Work out the finished part from the listing and answer in its coordinate system (mm). A direction names the side the tool comes from. Round coordinates to 2 decimals unless told otherwise and drop trailing zeros. Write each loop counter-clockwise with the first axis right and the second up, starting at its lowest first coordinate (ties: lowest second). Pieces come first, ordered by that corner, then holes. Notation, with made-up numbers: (49.25, -32.5) -> (55.25, -32.5) arc R19 ccw to (55.25, 2.5) -> close; hole circle Ø10 at (-5, -39.75). An arc over 180 degrees is marked (long way). One line per item, written item: value.
```python
from build123d import *

# Parameters (mm, degrees)
F0_W         = 25.3122672439
F0_H         = 26.0148867965
F1_DEPTH     = 30
F2_W         = 13.9388088137
F2_H         = 14.6495383233
F3_DEPTH     = 32
F4_T1_DEPTH  = 18.0148867965
F4_T3_DEPTH  = 31.3122672439
F4_T5_DEPTH  = 36
F4_T7_DEPTH  = 22
F4_T9_DEPTH  = 50
F4_T11_DEPTH = 32.0148867965
F4_S15_W     = 4
F4_S15_H     = 4
F4_T16_DEPTH = 4
F4_S21_W     = 4
F4_S21_H     = 4
F4_T22_DEPTH = 4
F4_S27_W     = 4
F4_S27_H     = 4
F4_T28_DEPTH = 4
F5_T1_DEPTH  = 31.3122672439
F5_S5_W      = 4
F5_S5_H      = 4
F5_T6_DEPTH  = 4


# Not quite as in the source:
# - a fillet or chamfer that OpenCascade refuses, or shapes differently, is made with other operations: its cross-section is extruded or revolved along the edge and cut away or added


with BuildPart() as f1:
    # F0 (on Front) → F1 (new body)
    with BuildSketch(Plane.XZ):
        with Locations((12.6561336219, 13.0074433982)):
            Rectangle(F0_W, F0_H)
    extrude(amount=F1_DEPTH)

    # F2 (on face) → F3 (cut)
    with BuildSketch(Plane(origin=(0, 0, 0), x_dir=(-1, 0, 0), z_dir=(0, 1, 0))):
        with Locations((-9.6562495455, 15.7833071426)):
            Rectangle(F2_W, F2_H)
    extrude(amount=-F3_DEPTH, mode=Mode.SUBTRACT)

    # F4: fillet of radius 4 on 8 edges, made by hand

    # F4_s2 → F4_t1 (cut)
    with BuildSketch(Plane.XY.offset(4)):
        with BuildLine():
            ThreePointArc((21.3122672439, -30), (24.1406943686, -28.8284271247), (25.3122672439, -26))
            Line((25.3122672439, -26), (25.3122672439, -30))
            Line((25.3122672439, -30), (21.3122672439, -30))
        make_face()
    extrude(amount=F4_T1_DEPTH, mode=Mode.SUBTRACT)

    # F4_s4 → F4_t3 (cut)
    with BuildSketch(Plane.YZ.offset(-10)):
        with BuildLine():
            ThreePointArc((-26, 26.0148867965), (-28.8284271247, 24.8433139212), (-30, 22.0148867965))
            Line((-30, 22.0148867965), (-30, 26.0148867965))
            Line((-30, 26.0148867965), (-26, 26.0148867965))
        make_face()
        with BuildLine():
            ThreePointArc((-26, 0), (-28.8284271247, 1.1715728753), (-30, 4))
            Line((-30, 4), (-30, 0))
            Line((-30, 0), (-26, 0))
        make_face()
        with BuildLine():
            ThreePointArc((-4, 26.0148867965), (-1.1715728753, 24.8433139212), (0, 22.0148867965))
            Line((0, 22.0148867965), (0, 26.0148867965))
            Line((0, 26.0148867965), (-4, 26.0148867965))
        make_face()
    extrude(amount=F4_T3_DEPTH, mode=Mode.SUBTRACT)

    # F4_s6 → F4_t5 (cut)
    with BuildSketch(Plane.XZ.offset(-10)):
        with BuildLine():
            ThreePointArc((21.3122672439, 0), (24.1406943686, 1.1715728753), (25.3122672439, 4))
            Line((25.3122672439, 4), (25.3122672439, 0))
            Line((25.3122672439, 0), (21.3122672439, 0))
        make_face()
    extrude(amount=F4_T5_DEPTH, mode=Mode.SUBTRACT)

    # F4_s8 → F4_t7 (cut)
    with BuildSketch(Plane.XZ.offset(4)):
        with BuildLine():
            ThreePointArc((21.3122672439, 26.0148867965), (24.1406943686, 24.8433139212), (25.3122672439, 22.0148867965))
            Line((25.3122672439, 22.0148867965), (25.3122672439, 26.0148867965))
            Line((25.3122672439, 26.0148867965), (21.3122672439, 26.0148867965))
        make_face()
    extrude(amount=F4_T7_DEPTH, mode=Mode.SUBTRACT)

    # F4_s10 → F4_t9 (cut)
    with BuildSketch(Plane.XZ.offset(-10)):
        with BuildLine():
            ThreePointArc((0, 22.0148867965), (1.1715728753, 24.8433139212), (4, 26.0148867965))
            Line((4, 26.0148867965), (0, 26.0148867965))
            Line((0, 26.0148867965), (0, 22.0148867965))
        make_face()
    extrude(amount=F4_T9_DEPTH, mode=Mode.SUBTRACT)

    # F4_s12 → F4_t11 (cut)
    with BuildSketch(Plane.XY.offset(-10)):
        with BuildLine():
            ThreePointArc((21.3122672439, 0), (24.1406943686, -1.1715728753), (25.3122672439, -4))
            Line((25.3122672439, -4), (25.3122672439, 0))
            Line((25.3122672439, 0), (21.3122672439, 0))
        make_face()
    extrude(amount=F4_T11_DEPTH, mode=Mode.SUBTRACT)


with BuildPart() as f4_tool14:
    # F4_s15 → F4_t16 (new body)
    with BuildSketch(Plane.XY.offset(4)):
        with Locations((23.3122672439, -28)):
            Rectangle(F4_S15_W, F4_S15_H)
    extrude(amount=-F4_T16_DEPTH)

    # F4_s17 → F4_t18 (revolve, cut)
    with BuildSketch(Plane(origin=(21.3122672439, -26, 4), x_dir=(-0.7071067812, 0.7071067812, 0), z_dir=(-0.7071067812, -0.7071067812, 0))):
        with BuildLine():
            ThreePointArc((0, -4), (4, 0), (0, 4))
            Line((0, 4), (0, -4))
        make_face()
    revolve(axis=Axis((21.3122672439, -26, 4), (0, 0, -1)), mode=Mode.SUBTRACT)


with BuildPart() as f1_1:
    add(f1.part)

    # F4_t13: cut F4_tool14
    add(f4_tool14.part, mode=Mode.SUBTRACT)


with BuildPart() as f4_tool20:
    # F4_s21 → F4_t22 (new body)
    with BuildSketch(Plane.XY.offset(22.0148867965)):
        with Locations((23.3122672439, -28)):
            Rectangle(F4_S21_W, F4_S21_H)
    extrude(amount=F4_T22_DEPTH)

    # F4_s23 → F4_t24 (revolve, cut)
    with BuildSketch(Plane(origin=(21.3122672439, -26, 22.0148867965), x_dir=(-0.7071067812, 0.7071067812, 0), z_dir=(0.7071067812, 0.7071067812, 0))):
        with BuildLine():
            ThreePointArc((0, -4), (4, 0), (0, 4))
            Line((0, 4), (0, -4))
        make_face()
    revolve(axis=Axis((21.3122672439, -26, 22.0148867965), (0, 0, 1)), mode=Mode.SUBTRACT)


with BuildPart() as f1_2:
    add(f1_1.part)

    # F4_t19: cut F4_tool20
    add(f4_tool20.part, mode=Mode.SUBTRACT)


with BuildPart() as f4_tool26:
    # F4_s27 → F4_t28 (new body)
    with BuildSketch(Plane.XY.offset(22.0148867965)):
        with Locations((23.3122672439, -2)):
            Rectangle(F4_S27_W, F4_S27_H)
    extrude(amount=F4_T28_DEPTH)

    # F4_s29 → F4_t30 (revolve, cut)
    with BuildSketch(Plane(origin=(21.3122672439, -4, 22.0148867965), x_dir=(-0.7071067812, -0.7071067812, 0), z_dir=(-0.7071067812, 0.7071067812, 0))):
        with BuildLine():
            ThreePointArc((0, -4), (4, 0), (0, 4))
            Line((0, 4), (0, -4))
        make_face()
    revolve(axis=Axis((21.3122672439, -4, 22.0148867965), (0, 0, 1)), mode=Mode.SUBTRACT)


with BuildPart() as f1_3:
    add(f1_2.part)

    # F4_t25: cut F4_tool26
    add(f4_tool26.part, mode=Mode.SUBTRACT)

    # F5: fillet of radius 4 on 1 edges, made by hand

    # F5_s2 → F5_t1 (cut)
    with BuildSketch(Plane.YZ.offset(-10)):
        with BuildLine():
            ThreePointArc((0, 4), (-1.1715728753, 1.1715728753), (-4, 0))
            Line((-4, 0), (0, 0))
            Line((0, 0), (0, 4))
        make_face()
    extrude(amount=F5_T1_DEPTH, mode=Mode.SUBTRACT)


with BuildPart() as f5_tool4:
    # F5_s5 → F5_t6 (new body)
    with BuildSketch(Plane.XZ.offset(4)):
        with Locations((23.3122672439, 2)):
            Rectangle(F5_S5_W, F5_S5_H)
    extrude(amount=-F5_T6_DEPTH)

    # F5_s7 → F5_t8 (revolve, cut)
    with BuildSketch(Plane(origin=(21.3122672439, -4, 4), x_dir=(-0.7071067812, 0, 0.7071067812), z_dir=(-0.7071067812, 0, -0.7071067812))):
        with BuildLine():
            ThreePointArc((0, -4), (4, 0), (0, 4))
            Line((0, 4), (0, -4))
        make_face()
    revolve(axis=Axis((21.3122672439, -4, 4), (0, 1, 0)), mode=Mode.SUBTRACT)


with BuildPart() as f1_4:
    add(f1_3.part)

    # F5_t3: cut F5_tool4
    add(f5_tool4.part, mode=Mode.SUBTRACT)


solid = f1_4.part
```
(1) Consider probe 1 along Z at (x, y) = (5.5, -25.5); probe 2 along X at (y, z) = (-14.25, 13.75); probe 3 along Z at (x, y) = (5.75, -3.25). Determine where each line is inside the solid, lowest interval first.
Reported:
probe 1: z = 0 to 8.46, 23.11 to 26.01
probe 2: x = 0 to 2.69, 16.63 to 25.31
probe 3: z = 0.07 to 8.46, 23.11 to 25.94
(2) For a pull along X with two mould halves and no side action, classify faces 3 (the face through (13, 0, 7)), 4 (the face through (10, -15, 8.459)), 5 (the face through (1.14, -14.79, 24.81)), 6 (the face through (24.109, -14.846, 24.874)) as pulls with the +X half, pulls with the -X half, needs draft (parallel to the pull), parting line crosses it, or undercut.
Reported:
face 3: needs draft
face 4: undercut
face 5: pulls with the -X half
face 6: pulls with the +X half
(3) Find section C-C on y = -8. Give the vertices of the cut face in (x, z), plus the area to 3 significant figures.
Reported:
outline: (0, 0) -> (21.31, 0) arc R4 ccw to (25.31, 4) -> (25.31, 22.01) arc R4 ccw to (21.31, 26.01) -> (4, 26.01) arc R4 ccw to (0, 22.01) -> close; hole (2.69, 8.46) -> (16.63, 8.46) -> (16.63, 23.11) -> (2.69, 23.11) -> close
area: 444 mm2
(4) Find section D-D on z = 24. Give the vertices of the cut face in (x, y), plus the area to 3 significant figures.
Reported:
outline: (0.53, -29.47) -> (21.31, -29.47) arc R3.47 ccw to (24.78, -26) -> (24.78, -4) arc R3.47 ccw to (21.31, -0.53) -> (0.53, -0.53) -> close
area: 697 mm2
(5) Find section A-A on x = 7. Give the vertices of the cut face in (y, z), plus the area to 3 significant figures.
Reported:
outline: (-30, 4) arc R4 ccw to (-26, 0) -> (-4, 0) arc R4 ccw to (0, 4) -> (0, 8.46) -> (-30, 8.46) -> close; (-29.85, 23.11) -> (-0.15, 23.11) arc R4 ccw to (-4, 26.01) -> (-26, 26.01) arc R4 ccw to start
area: 327 mm2
(6) Find section B-B on z = 17.5. Give the vertices of the cut face in (x, y), plus the area to 3 significant figures.
Reported:
outline: (0, -30) -> (2.69, -30) -> (2.69, 0) -> (0, 0) -> close; (16.63, -30) -> (21.31, -30) arc R4 ccw to (25.31, -26) -> (25.31, -4) arc R4 ccw to (21.31, 0) -> (16.63, 0) -> close
area: 334 mm2
(7) A tool of negligible diameter and unlimited length cuts with its end or side. For faces 1 (the face through (25.312, -15, 13)), 2 (the face through (2.687, -15, 16)), from which of +Z, -Z, +X, -X, +Y, -Y can it reach the whole face along a straight path? Write none if from no direction.
Reported:
face 1: +Z, -Z, +X, +Y, -Y
face 2: +Y, -Y
(8) Flat-ended cylindrical pins translate along their axes: pin 1 Ø5 at (x, z) = (7.5, 12.5) entering from -Y; pin 2 Ø1.5 at (x, z) = (17, 3) entering from +Y. Find the tip coordinate at first contact, or state that the pin passes through.
Reported:
pin 1: passes through
pin 2: stops at y = -0.01
